```python
from build123d import *

# Parameters (mm, degrees)
CROQUIS1_R                          = 13
CROQUIS1_R_2                        = 11.05
SALIENTE_EXTRUIR1_DEPTH             = 1
BARRER_L_MINA1_PROFILE_R            = 13.05
BARRER_L_MINA1_PROFILE_R_2          = 11.05
CROQUIS19_R                         = 13
CROQUIS19_R_2                       = 11.05
SALIENTE_EXTRUIR2_DEPTH             = 14
SALIENTE_EXTRUIR2_DIRECTION_2_REACH = 72.145
CORTAR_EXTRUIR1_REACH               = 78.822
CROQUIS20_R                         = 11.05


with BuildPart() as part:
    # Croquis1 → Saliente-Extruir1 (new body)
    with BuildSketch(Plane(origin=(0, 0, 0), x_dir=(1, 0, 0), z_dir=(0, 1, 0))):
        with Locations(Location((0, 0, 0), (0, 0, 270))):
            Circle(CROQUIS1_R)
        with Locations(Location((0, 0, 0), (0, 0, 270))):
            Circle(CROQUIS1_R_2, mode=Mode.SUBTRACT)
    extrude(amount=SALIENTE_EXTRUIR1_DEPTH)

    # Barrer-L_mina1: sweep along a path in Croquis2
    with BuildLine(Plane.XY) as barrer_l_mina1_path:
        Line((0, 1), (0, 21))
        ThreePointArc((0, 21), (-2.727754239, 29.625078781), (-9.918931196, 35.113211534))
        Line((-9.918931196, 35.113211534), (-29.677427344, 42.226707859))
    # Barrer-L_mina1 profile (on start of the path) → Barrer-L_mina1 (sweep)
    with BuildSketch(Plane.ZX.offset(1)):
        Circle(BARRER_L_MINA1_PROFILE_R)
        Circle(BARRER_L_MINA1_PROFILE_R_2, mode=Mode.SUBTRACT)
    sweep(path=barrer_l_mina1_path.line)

    # Croquis19 → Saliente-Extruir2 (add)
    with BuildSketch(Plane.XY.offset(15)):
        with Locations((0, 13)):
            Circle(CROQUIS19_R)
        with Locations((0, 13)):
            Circle(CROQUIS19_R_2, mode=Mode.SUBTRACT)
    extrude(amount=SALIENTE_EXTRUIR2_DEPTH)

    # Croquis19 → Saliente-Extruir2 direction 2 (add, up to next)
    with BuildSketch(Plane.XY.offset(15), mode=Mode.PRIVATE) as saliente_extruir2_direction_2_sk1:
        with Locations((0, 13)):
            Circle(CROQUIS19_R)
        with Locations((0, 13)):
            Circle(CROQUIS19_R_2, mode=Mode.SUBTRACT)
    saliente_extruir2_direction_2_tool1 = extrude(saliente_extruir2_direction_2_sk1.sketch, amount=-SALIENTE_EXTRUIR2_DIRECTION_2_REACH, mode=Mode.PRIVATE) - part.part
    add(saliente_extruir2_direction_2_tool1.solids().sort_by_distance((-12.632304, 13, 15))[0])

    # Croquis20 → Cortar-Extruir1 (cut, up to next)
    with BuildSketch(Plane.XY.offset(29), mode=Mode.PRIVATE) as cortar_extruir1_sk1:
        with Locations((0, 13)):
            Circle(CROQUIS20_R)
    cortar_extruir1_tool1 = extrude(cortar_extruir1_sk1.sketch, amount=-CORTAR_EXTRUIR1_REACH, mode=Mode.PRIVATE) & part.part
    add(cortar_extruir1_tool1.solids().sort_by_distance((0, 13, 29))[0], mode=Mode.SUBTRACT)


solid = part.part
```
Here's how the part is built. I have some questions about the finished solid (model axes, mm). A direction names the side the tool comes from. Coordinates: 2 decimals unless noted, no trailing zeros. Order: outer loops, then holes, each group sorted by start corner. A loop starts at its lowest first (then second) coordinate and runs counter-clockwise, first axis right, second up. Notation, with made-up numbers: M -22.5,-35.75 L 28.5,-35.75 A17 cw 28.5,-31.75 Z; hole C 43,65 d4. An arc over 180 degrees is marked long. Answer as a JSON object with one key per item and string values. Group by question number.
(1) Suppose I cut it at C-C, the plane z = 10. Please give me the cut outline in (x, y), then the cut area to 3 significant figures.
(2) Suppose I cut it at B-B, the plane z = -9.5. Please give me the cut outline in (x, y), then the cut area to 3 significant figures.
(3) I need wall thicknesses on probe 1 along X at (y, z) = (6.75, 0); probe 2 along Y at (x, z) = (0, 17.5). Which ranges of each line are inside material? Lowest first, please.
(4) For pin 1 (6 mm diameter, centred on x = -14.5, z = 9.5, fed in from -Y); pin 2 (10 mm diameter, centred on x = -18, z = -1, fed in from +Y); pin 3 (10 mm diameter, centred on y = 7.5, z = 7.5, fed in from +X), each with a flat end and sliding along its axis, tell me the tip position at first contact or that it passes through.
(5) Which directions (+Z, -Z, +X, -X, +Y, -Y) give clear straight access to the entire face, cutting with the end or side of a thin tool? Please do faces 1 (the face through (-11.04, 13.49, 17.52)), 2 (the face through (-10, 0, -6)), 3 (the face through (0.49, 10.35, -11.04)).
(6) If we mould it in two halves opening along X, with no side actions, what happens to faces 4 (the face through (-12.987, 13.572, 18.36)), 5 (the face through (-26.38, 51.38, 5.86)), 6 (the face through (-23.26, 29.5, 5.1))? For each: released by +X, released by -X, zero draft, split by the parting line, or undercut.
Values found:
{
 "1": {"outline": "M -32.52,34.34 L -12.76,27.22 A6.62 cw -8.62,22.73 A13 ccw -8.38,3.07 L -8.38,1 L -8.31,1 L -8.31,0 L -4.7,0 L -4.7,3 A11.05 cw -4.88,22.91 A10.3 ccw -11.51,30.69 L -31.27,37.8 Z; M -28.08,46.65 L -8.33,39.54 A19.7 cw 4.59,23.05 A11.05 cw 4.7,3 L 4.7,0 L 8.31,0 L 8.31,1 L 8.38,1 L 8.38,3.07 A13 ccw 8.3,23.01 A23.38 ccw -7.08,43 L -26.84,50.12 Z", "area": "390 mm^2"},
 "2": {"outline": "M -32.71,33.81 L -12.95,26.69 A6.05 cw -8.95,21 L -8.95,1 L -8.87,1 L -8.87,0 L -5.64,0 L -5.64,21 A9.36 ccw -11.83,29.8 L -31.59,36.92 Z; M -27.77,47.54 L -8.01,40.42 A20.64 cw 5.64,21 L 5.64,0 L 8.87,0 L 8.87,1 L 8.95,1 L 8.95,21 A23.95 ccw -6.89,43.53 L -26.65,50.64 Z", "area": "399 mm^2"},
 "3": {"probe 1": "x = -13.05 to -11.05, 11.05 to 13.05", "probe 2": "y = 0 to 1.95, 24.05 to 26"},
 "4": {"pin 1": "stops at y = 6.94", "pin 2": "stops at y = 53.67", "pin 3": "stops at x = 12.99"},
 "5": {"face 1": "+Z", "face 2": "+Z, -Z, +X, -X, -Y", "face 3": "-Y"},
 "6": {"face 4": "split by the parting line", "face 5": "released by -X", "face 6": "undercut"}
}
